```python
from build123d import *

# Parameters (mm, degrees)
BOSS_EXTRUDE1_DEPTH     = 10
SKETCH3_W               = 110
SKETCH3_H               = 6.65
SKETCH4_W               = 18
SKETCH4_H               = 18
BOSS_EXTRUDE2_DEPTH     = 10
SKETCH5_W               = 10
SKETCH5_H               = 10
CUT_EXTRUDE1_DEPTH      = 10
CUT_EXTRUDE1_DEPTH_BACK = 10
HOLE1_D                 = 4.134
HOLE1_DEPTH             = 9
HOLE1_CSINK_D           = 5
HOLE1_CSINK_ANGLE       = 90
HOLE2_D                 = 4.134
HOLE2_DEPTH             = 11
HOLE2_CSINK_D           = 5
HOLE2_CSINK_ANGLE       = 90
HOLE2_TIP               = 1.193383006


with BuildPart() as part:
    # Sketch1 → Revolve1 (revolve)
    with BuildSketch(Plane.XY, mode=Mode.PRIVATE) as revolve1_sk:
        with BuildLine():
            Line((0, 0), (0, 7))
            Line((0, 7), (1, 8))
            Line((1, 8), (11.95, 8))
            Line((11.95, 8), (12.865685425, 7.084314575))
            ThreePointArc((12.865685425, 7.084314575), (13.125224104, 6.910896374), (13.43137085, 6.85))
            Line((13.43137085, 6.85), (14.2, 6.85))
            ThreePointArc((14.2, 6.85), (14.765685425, 7.084314575), (15, 7.65))
            Line((15, 7.65), (15, 8))
            Line((15, 8), (17, 8))
            Line((17, 8), (17, 0))
            Line((17, 0), (0, 0))
        make_face()
    revolve(revolve1_sk.sketch.rotate(Axis((17, 0, 0), (-1, 0, 0)), 270), axis=Axis((17, 0, 0), (-1, 0, 0)))

    # Sketch2 → Boss-Extrude1 (add)
    with BuildSketch(Plane(origin=(17, 0, 0), x_dir=(0, 0, -1), z_dir=(1, 0, 0))):
        with BuildLine():
            Line((-4.358898944, -9), (4.358898944, -9))
            ThreePointArc((4.358898944, -9), (7.071067812, -7.071067812), (9, -4.358898944))
            Line((9, -4.358898944), (9, 4.358898944))
            ThreePointArc((9, 4.358898944), (7.071067812, 7.071067812), (4.358898944, 9))
            Line((4.358898944, 9), (-4.358898944, 9))
            ThreePointArc((-4.358898944, 9), (-7.071067812, 7.071067812), (-9, 4.358898944))
            Line((-9, 4.358898944), (-9, -4.358898944))
            ThreePointArc((-9, -4.358898944), (-7.071067812, -7.071067812), (-4.358898944, -9))
        make_face()
    extrude(amount=BOSS_EXTRUDE1_DEPTH)

    # Sketch3 → Revolve2 (revolve)
    with BuildSketch(Plane.XY, mode=Mode.PRIVATE) as revolve2_sk:
        with Locations((82, 3.325)):
            Rectangle(SKETCH3_W, SKETCH3_H)
    revolve(revolve2_sk.sketch.rotate(Axis((137, 0, 0), (-1, 0, 0)), 270), axis=Axis((137, 0, 0), (-1, 0, 0)))

    # Sketch4 → Boss-Extrude2 (add)
    with BuildSketch(Plane(origin=(137, 0, 0), x_dir=(0, 0, -1), z_dir=(1, 0, 0))):
        Rectangle(SKETCH4_W, SKETCH4_H)
    extrude(amount=BOSS_EXTRUDE2_DEPTH)

    # Sketch5 → Cut-Revolve1 (revolve, cut)
    with BuildSketch(Plane.XY):
        with Locations((142, 15)):
            Rectangle(SKETCH5_W, SKETCH5_H)
    revolve(axis=Axis((147, 0, 0), (-1, 0, 0)), mode=Mode.SUBTRACT)

    # Sketch6 → Revolve3 (revolve)
    with BuildSketch(Plane.XY, mode=Mode.PRIVATE) as revolve3_sk:
        with BuildLine():
            Line((147, 0), (147, 8))
            Line((147, 8), (149, 8))
            Line((149, 8), (149, 7.65))
            ThreePointArc((149, 7.65), (149.234314575, 7.084314575), (149.8, 6.85))
            Line((149.8, 6.85), (150.56862915, 6.85))
            ThreePointArc((150.56862915, 6.85), (150.874775896, 6.910896374), (151.134314575, 7.084314575))
            Line((151.134314575, 7.084314575), (152.05, 8))
            Line((152.05, 8), (163, 8))
            Line((163, 8), (164, 7))
            Line((164, 7), (164, 0))
            Line((164, 0), (147, 0))
        make_face()
    revolve(revolve3_sk.sketch.rotate(Axis((164, 0, 0), (-1, 0, 0)), 270), axis=Axis((164, 0, 0), (-1, 0, 0)))

    # Sketch7 → Cut-Extrude1 (cut, two sides: drawn at the far end of the back side and taken through both)
    with BuildSketch(Plane(origin=(0, 0, 0), x_dir=(1, 0, 0), z_dir=(0, 1, 0)).offset(-CUT_EXTRUDE1_DEPTH_BACK)):
        Polygon((141, 18), (141, 6), (164, 6), (164, -6), (141, -6), (141, -18), (176, -18), (176, 18), align=None)
    extrude(amount=CUT_EXTRUDE1_DEPTH + CUT_EXTRUDE1_DEPTH_BACK, mode=Mode.SUBTRACT)

    # Sketch8 → Cut-Revolve2 (revolve, cut)
    with BuildSketch(Plane(origin=(150, 0, 0), x_dir=(0, 0, -1), z_dir=(1, 0, 0)), mode=Mode.PRIVATE) as cut_revolve2_sk:
        Polygon((-6.2, 0), (-6.2, 4.692820323), (-5, 4), (-4.5, 4), (-5, 3.711324865), (-5, 3), (5, 3), (5, 3.711324865), (4.5, 4), (5, 4), (6.2, 4.692820323), (6.2, 0), align=None)
    revolve(cut_revolve2_sk.sketch.rotate(Axis((150, 0, -5), (0, 0, 1)), 270), axis=Axis((150, 0, -5), (0, 0, 1)), mode=Mode.SUBTRACT)

    # Hole1
    with Locations(Plane(origin=(0, 9, 0), x_dir=(1, 0, 0), z_dir=(0, 1, 0))):
        with Locations((23, 0)):
            CounterSinkHole(HOLE1_D / 2, HOLE1_CSINK_D / 2, depth=HOLE1_DEPTH, counter_sink_angle=HOLE1_CSINK_ANGLE)

    # Hole2
    with Locations(Plane(origin=(0, 9, 0), x_dir=(1, 0, 0), z_dir=(0, 1, 0))):
        with Locations((141, 0)):
            CounterSinkHole(HOLE2_D / 2, HOLE2_CSINK_D / 2, depth=HOLE2_DEPTH, counter_sink_angle=HOLE2_CSINK_ANGLE)
            with Locations((0, 0, -(HOLE2_DEPTH + HOLE2_TIP / 2))):  # 120° drill point
                Cone(0, HOLE2_D / 2, HOLE2_TIP, mode=Mode.SUBTRACT)

    # Sketch13 → Cut-Revolve3 (revolve, cut)
    with BuildSketch(Plane.XY, mode=Mode.PRIVATE) as cut_revolve3_sk:
        Polygon((-5, 0), (-5, 3), (37.3, 3), (37.3, 6), (120.3, 6), (120.3, 0), align=None)
    revolve(cut_revolve3_sk.sketch.rotate(Axis((120.3, 0, 0), (-1, 0, 0)), 270), axis=Axis((120.3, 0, 0), (-1, 0, 0)), mode=Mode.SUBTRACT)


solid = part.part
```
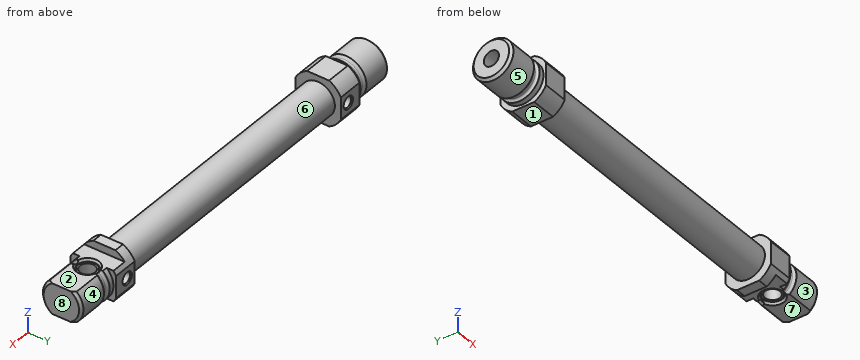
The listing builds one solid part. Answer for the finished solid, in the listing's coordinates (mm). Face numbers are marked on the shaded views. A direction names the side the tool comes from. Coordinates: 2 decimals unless noted, no trailing zeros. Write each loop counter-clockwise with the first axis right and the second up, starting at its lowest first coordinate (ties: lowest second). Pieces come first, ordered by that corner, then holes. Notation, with made-up numbers: (-1, 18) -> (48, 18) arc R12 cw to (48, 35) -> close; hole circle Ø9 at (-34, 7.5). An arc over 180 degrees is marked (long way). Write each question's results on one line, items separated by ' | '. Start each with the question number.
1) A cutting plane is placed at D-D (x = 134). Determine the outline of the cut face in (y, z), then the cut area to 3 significant figures.
2) Flat-ended cylindrical pins translate along their axes: pin 1 Ø6 at (y, z) = (-2.5, 0.5) entering from -X; pin 2 Ø8 at (x, z) = (37, -1.5) entering from -Y; pin 3 Ø10 at (x, y) = (59, 4) entering from -Z; pin 4 Ø3.5 at (x, y) = (151.5, 0.5) entering from -Z. Find the tip coordinate at first contact, or state that the pin passes through.
3) For a pull along X with two mould halves and no side action, classify the marked faces 6, 7 and 8 as +X half, -X half, draft (parallel to the pull), parting line (faces both ways), or undercut.
4) A tool of negligible diameter and unlimited length cuts with its end or side. For the marked faces 1, 2, 3, 4 and 5, from which of +Z, -Z, +X, -X, +Y, -Y can it reach the whole face along a straight path? Write none if from no direction.
5) A cutting plane is placed at A-A (x = 23). Determine the outline of the cut face in (y, z).
6) A cutting plane is placed at B-B (y = 0). Count the separate pieces of the cut face and the enclosed holes in it, then the cut area to 3 significant figures.
7) Straight lines are drawn through the part: probe 1 along X at (y, z) = (7, -7); probe 2 along Y at (x, z) = (29, 0); probe 3 along X at (y, z) = (-1.5, 1). For each, find the intervals that lie inside material, in ascending order.
8) A cutting plane is placed at C-C (x = 115). Determine the outline of the cut face in (y, z).
Values follow:
1) outline: circle Ø13.3 at (0, 0) | area: 139 mm²
2) pin 1: x = 0 | pin 2: y = -6.65 | pin 3: z = -6.65 | pin 4: z = -5
3) face 6: undercut | face 7: draft | face 8: +X half
4) face 1: -Z, +X, -X, +Y, -Y | face 2: +Z, +X, +Y, -Y | face 3: +X, -Y | face 4: +X, +Y | face 5: -X
5) outline: (-9, -4.36) arc R10 ccw to (-4.36, -9) -> (4.36, -9) arc R10 ccw to (9, -4.36) -> (9, -2.5) -> (8.57, -2.07) -> (2.17, -2.07) arc R3 cw (long way) to (2.17, 2.07) -> (8.57, 2.07) -> (9, 2.5) -> (9, 4.36) arc R10 ccw to (4.36, 9) -> (-4.36, 9) arc R10 ccw to (-9, 4.36) -> close
6) separate pieces: 2 | enclosed holes: 1 | area: 946 mm²
7) probe 1: 17 to 27, 137 to 141 | probe 2: -6.65 to -3, 3 to 6.65 | probe 3: 120.3 to 139.19, 142.81 to 147.4, 152.6 to 164
8) outline: circle Ø13.3 at (0, 0); hole circle Ø12 at (0, 0)
